The model under review builds one solid part; all positions refer to its coordinate system, in mm. A direction names the side the tool comes from. Round coordinates to 2 decimals unless told otherwise and drop trailing zeros. Write each loop counter-clockwise with the first axis right and the second up, starting at its lowest first coordinate (ties: lowest second). Pieces come first, ordered by that corner, then holes. Notation, with made-up numbers: M 48.5,58.5 L 85.5,58.5 A12 cw 85.5,70.5 Z; hole C 13,10.5 d11. An arc over 180 degrees is marked long. One line per item, written item: value. Start each with the question number.
1) Mouldability with a two-part tool opening along X and no side actions: class faces 1 (the face through (351.4, 6.07, -1.14)), 2 (the face through (342.706, 31.434, -2.694)), 3 (the face through (337.85, 61.43, 0.6)) as +X half, -X half, draft (parallel to the pull), parting line (faces both ways), or undercut.
2) Take a section at C-C, the plane x = 353. Write out the cut boundary in (y, z), and give its area (3 significant figures).
3) Wall thickness on probe 1 along Y at (x, z) = (359.5, -1.2); probe 2 along Y at (x, z) = (322, -2.25); probe 3 along X at (y, z) = (48.5, -0.65): over which ranges is each line inside the solid? List them lowest first.
4) Take a section at B-B, the plane y = 13.5. Write out the cut boundary in (x, z), and give its area (3 significant figures).
5) Tool access review of faces 4 (the face through (326.07, 50.5, -1.85)), 5 (the face through (312.5, 59, -2)), 6 (the face through (337.85, 0.57, 0.6)): name each direction out of +Z, -Z, +X, -X, +Y, -Y from which nothing blocks a thin tool from reaching the whole face with its end or side.
6) For P1, Ø3.5, axis at x = 359.5, y = 13.5, coming from the -Z side; P2, Ø1, axis at y = 28, z = -1.5, coming from the -X side; P3, Ø15, axis at x = 346, y = 42.5, coming from the +Z side; P4, Ø3, axis at x = 353, y = 6, coming from the +Z side, all flat-tipped, find the tip position at first contact; note any pin that passes through.
7) Take a section at D-D, the plane y = 36. Write out the cut boundary in (x, z).
8) Take a section at A-A, the plane z = -0.75. State how many separate pieces and enclosed holes the cut face has, and give its area (3 significant figures).
from build123d import *

# Parameters (mm, degrees)
CYLINDER138_R          = 1.6
CYLINDER138_DEPTH      = 10
CYLINDER139_R          = 1.6
CYLINDER139_DEPTH      = 10
CYLINDER140_R          = 1.6
CYLINDER140_DEPTH      = 10
CYLINDER141_R          = 1.6
CYLINDER141_DEPTH      = 10
BOX063_W               = 62
BOX063_H               = 10
BOX063_DEPTH           = 29
BOX064_W               = 62
BOX064_H               = 10
BOX064_DEPTH           = 29
CYLINDER103_R          = 1.6
CYLINDER103_DEPTH      = 10
CYLINDER102_R          = 1.6
CYLINDER102_DEPTH      = 10
CYLINDER104_R          = 1.6
CYLINDER104_DEPTH      = 10
CYLINDER105_R          = 1.6
CYLINDER105_DEPTH      = 10
CYLINDER099_R          = 1.6
CYLINDER099_DEPTH      = 15
CYLINDER098_R          = 1.6
CYLINDER098_DEPTH      = 15
CYLINDER101_R          = 1.6
CYLINDER101_DEPTH      = 15
CYLINDER100_R          = 1.6
CYLINDER100_DEPTH      = 15
BOX047_W               = 15
BOX047_H               = 42
BOX047_DEPTH           = 20
BOX046_W               = 50
BOX046_H               = 62
BOX046_DEPTH           = 20
FILLET018_R            = 2
BOX044_W               = 58
BOX044_H               = 68
BOX044_DEPTH           = 10
BOX044_PLACEMENT_ANGLE = 3
BOX045_W               = 50
BOX045_H               = 68
BOX045_DEPTH           = 22
FILLET019_R            = 5
FILLET020_R            = 2
FILLET021_R            = 5
FILLET022_R            = 3


with BuildPart() as cylinder138:
    # Cylinder138 → Cylinder138 (new body)
    with BuildSketch(Plane(origin=(320, 6, -6), x_dir=(1, 0, 0), z_dir=(0, 0, 1))):
        Circle(CYLINDER138_R)
    extrude(amount=CYLINDER138_DEPTH)


with BuildPart() as fusion116:
    # Cylinder139 → Cylinder139 (new body)
    with BuildSketch(Plane(origin=(320, 56, -6), x_dir=(1, 0, 0), z_dir=(0, 0, 1))):
        Circle(CYLINDER139_R)
    extrude(amount=CYLINDER139_DEPTH)

    # Fusion116: union Cylinder138
    add(cylinder138.part)


with BuildPart() as fusion116_1:
    # Fusion116 placement: moved
    add(fusion116.part.moved(Location((2, 0, 0))))


with BuildPart() as cylinder140:
    # Cylinder140 → Cylinder140 (new body)
    with BuildSketch(Plane(origin=(320, 6, -6), x_dir=(1, 0, 0), z_dir=(0, 0, 1))):
        Circle(CYLINDER140_R)
    extrude(amount=CYLINDER140_DEPTH)


with BuildPart() as fusion118:
    # Cylinder141 → Cylinder141 (new body)
    with BuildSketch(Plane(origin=(320, 56, -6), x_dir=(1, 0, 0), z_dir=(0, 0, 1))):
        Circle(CYLINDER141_R)
    extrude(amount=CYLINDER141_DEPTH)

    # Fusion117: union Cylinder140
    add(cylinder140.part)


with BuildPart() as fusion118_1:
    # Fusion117 placement: moved
    add(fusion118.part.moved(Location((33, 0, 0))))

    # Fusion118: union Fusion116
    add(fusion116_1.part)


with BuildPart() as cube042:
    # Box063 → Box063 (new body)
    with BuildSketch(Plane(origin=(309, -10, -9), x_dir=(1, 0, 0), z_dir=(0, 0, 1))):
        with Locations((31, 5)):
            Rectangle(BOX063_W, BOX063_H)
    extrude(amount=BOX063_DEPTH)


with BuildPart() as fusion115:
    # Box064 → Box064 (new body)
    with BuildSketch(Plane(origin=(309, 62, -9), x_dir=(1, 0, 0), z_dir=(0, 0, 1))):
        with Locations((31, 5)):
            Rectangle(BOX064_W, BOX064_H)
    extrude(amount=BOX064_DEPTH)

    # Fusion115: union Cube042
    add(cube042.part)


with BuildPart() as cylinder103:
    # Cylinder103 → Cylinder103 (new body)
    with BuildSketch(Plane(origin=(355, 7, 10), x_dir=(1, 0, 0), z_dir=(0, -1, 0))):
        Circle(CYLINDER103_R)
    extrude(amount=CYLINDER103_DEPTH)


with BuildPart() as fusion089:
    # Cylinder102 → Cylinder102 (new body)
    with BuildSketch(Plane(origin=(320, 7, 10), x_dir=(1, 0, 0), z_dir=(0, -1, 0))):
        Circle(CYLINDER102_R)
    extrude(amount=CYLINDER102_DEPTH)

    # Fusion089: union Cylinder103
    add(cylinder103.part)


with BuildPart() as cylinder104:
    # Cylinder104 → Cylinder104 (new body)
    with BuildSketch(Plane(origin=(355, 7, 10), x_dir=(1, 0, 0), z_dir=(0, -1, 0))):
        Circle(CYLINDER104_R)
    extrude(amount=CYLINDER104_DEPTH)


with BuildPart() as fusion091:
    # Cylinder105 → Cylinder105 (new body)
    with BuildSketch(Plane(origin=(320, 7, 10), x_dir=(1, 0, 0), z_dir=(0, -1, 0))):
        Circle(CYLINDER105_R)
    extrude(amount=CYLINDER105_DEPTH)

    # Fusion090: union Cylinder104
    add(cylinder104.part)


with BuildPart() as fusion091_1:
    # Fusion090 placement: moved
    add(fusion091.part.moved(Location((0, 58, 0))))

    # Fusion091: union Fusion089
    add(fusion089.part)


with BuildPart() as cylinder099:
    # Cylinder099 → Cylinder099 (new body)
    with BuildSketch(Plane(origin=(359.5, 13.5, -15), x_dir=(1, 0, 0), z_dir=(0, 0, 1))):
        Circle(CYLINDER099_R)
    extrude(amount=CYLINDER099_DEPTH)


with BuildPart() as fusion083:
    # Cylinder098 → Cylinder098 (new body)
    with BuildSketch(Plane(origin=(330.5, 13.5, -15), x_dir=(1, 0, 0), z_dir=(0, 0, 1))):
        Circle(CYLINDER098_R)
    extrude(amount=CYLINDER098_DEPTH)

    # Fusion083: union Cylinder099
    add(cylinder099.part)


with BuildPart() as cylinder101:
    # Cylinder101 → Cylinder101 (new body)
    with BuildSketch(Plane(origin=(359.5, 13.5, -15), x_dir=(1, 0, 0), z_dir=(0, 0, 1))):
        Circle(CYLINDER101_R)
    extrude(amount=CYLINDER101_DEPTH)


with BuildPart() as fusion085:
    # Cylinder100 → Cylinder100 (new body)
    with BuildSketch(Plane(origin=(330.5, 13.5, -15), x_dir=(1, 0, 0), z_dir=(0, 0, 1))):
        Circle(CYLINDER100_R)
    extrude(amount=CYLINDER100_DEPTH)

    # Fusion084: union Cylinder101
    add(cylinder101.part)


with BuildPart() as fusion085_1:
    # Fusion084 placement: moved
    add(fusion085.part.moved(Location((0, 35, 0))))

    # Fusion085: union Fusion083
    add(fusion083.part)


with BuildPart() as cube026:
    # Box047 → Box047 (new body)
    with BuildSketch(Plane(origin=(312.5, 10, -5), x_dir=(1, 0, 0), z_dir=(0, 0, 1))):
        with Locations((7.5, 21)):
            Rectangle(BOX047_W, BOX047_H)
    extrude(amount=BOX047_DEPTH)


with BuildPart() as fillet018:
    # Box046 → Box046 (new body)
    with BuildSketch(Plane(origin=(312.5, 0, 0), x_dir=(1, 0, 0), z_dir=(0, 0, 1))):
        with Locations((25, 31)):
            Rectangle(BOX046_W, BOX046_H)
    extrude(amount=BOX046_DEPTH)

    # Fillet018
    fillet018_edges = [fillet018.edges().sort_by_distance(p)[0] for p in [
        (337.5, 0, 0),
        (337.5, 62, 0),
    ]]
    fillet(fillet018_edges, radius=FILLET018_R)


with BuildPart() as cube023:
    # Box044 → Box044 (new body)
    with BuildSketch(Plane.XY):
        with Locations((29, 34)):
            Rectangle(BOX044_W, BOX044_H)
    extrude(amount=BOX044_DEPTH)


with BuildPart() as cube023_1:
    # Box044 placement: moved
    add(cube023.part.moved(Location((308.5, -3, -14.5))).rotate(Axis((308.5, -3, -14.5), (0, -1, 0)), BOX044_PLACEMENT_ANGLE))


with BuildPart() as battery_box_holder:
    # Box045 → Box045 (new body)
    with BuildSketch(Plane(origin=(312.5, -3, -5), x_dir=(1, 0, 0), z_dir=(0, 0, 1))):
        with Locations((25, 34)):
            Rectangle(BOX045_W, BOX045_H)
    extrude(amount=BOX045_DEPTH)

    # Cut051: cut Cube023
    add(cube023_1.part, mode=Mode.SUBTRACT)

    # Cut052: cut Fillet018
    add(fillet018.part, mode=Mode.SUBTRACT)

    # Cut053: cut Cube026
    add(cube026.part, mode=Mode.SUBTRACT)

    # Fillet019
    fillet019_edges = [battery_box_holder.edges().sort_by_distance(p)[0] for p in [
        (327.5, 10, -1.745264),
        (327.5, 52, -1.745264),
    ]]
    fillet(fillet019_edges, radius=FILLET019_R)

    # Fillet020
    fillet020_edges = [battery_box_holder.edges().sort_by_distance(p)[0] for p in [
        (337.5, -3, -2.966451),
        (337.5, 65, -2.966451),
    ]]
    fillet(fillet020_edges, radius=FILLET020_R)

    # Fillet021
    fillet021_edges = [battery_box_holder.edges().sort_by_distance(p)[0] for p in [
        (312.5, 10, -2.138323),
        (312.5, 52, -2.138323),
    ]]
    fillet(fillet021_edges, radius=FILLET021_R)

    # Cut054: cut Fusion085
    add(fusion085_1.part, mode=Mode.SUBTRACT)

    # Cut055: cut Fusion091
    add(fusion091_1.part, mode=Mode.SUBTRACT)

    # Fillet022
    fillet022_edges = [battery_box_holder.edges().sort_by_distance(p)[0] for p in [
        (312.5, -1.5, 17),
        (362.5, -1.5, 17),
        (362.5, 63.5, 17),
        (312.5, 63.5, 17),
    ]]
    fillet(fillet022_edges, radius=FILLET022_R)

    # Cut073: cut Fusion115
    add(fusion115.part, mode=Mode.SUBTRACT)

    # Cut074: cut Fusion118
    add(fusion118_1.part, mode=Mode.SUBTRACT)


solid = battery_box_holder.part
Checked values:
1. face 1: undercut
1. face 2: +X half
1. face 3: draft
2. outline: M 0,-2.15 L 4.4,-2.15 L 4.4,0 L 2,0 A2 cw 0,2 Z; M 7.6,-2.15 L 54.4,-2.15 L 54.4,0 L 7.6,0 Z; M 57.6,-2.15 L 62,-2.15 L 62,2 A2 cw 60,0 L 57.6,0 Z
2. area: 121 mm2
3. probe 1: y = 0 to 11.9, 15.1 to 46.9, 50.1 to 62
3. probe 2: y = 0 to 4.4, 7.6 to 10, 52 to 54.4, 57.6 to 62
3. probe 3: x = 327.27 to 328.9, 332.1 to 357.9, 361.1 to 362.5
4. outline: M 327.27,-3.5 L 328.9,-3.42 L 328.9,0 L 327.27,0 Z; M 332.1,-3.25 L 357.9,-1.9 L 357.9,0 L 332.1,0 Z; M 361.1,-1.73 L 362.5,-1.66 L 362.5,0 L 361.1,0 Z
4. area: 74.4 mm2
5. face 4: +Z, -Z, -X
5. face 5: +Z, -Z, -X, +Y, -Y
5. face 6: +Z, +X, -X
6. P1: stops at z = -1.91
6. P2: stops at x = 327.5
6. P3: stops at z = 0
6. P4: passes through
7. outline: M 327.5,-3.49 L 362.5,-1.66 L 362.5,0 L 327.5,0 Z
8. separate pieces: 1
8. enclosed holes: 8
8. area: 2,410 mm2
